from build123d import *

# Parameters (mm, degrees)
F0_R     = 1
F1_DEPTH = 8.3
F2_SIZE  = 0.5


with BuildPart() as f1:
    # F0 (on Top) → F1 (new body)
    with BuildSketch(Plane.XY):
        with BuildLine():
            Line((3.666061, 3.4), (-3.666061, 3.4))
            ThreePointArc((-3.666061, 3.4), (-5, 0), (-3.666061, -3.4))
            Line((-3.666061, -3.4), (3.666061, -3.4))
            ThreePointArc((3.666061, -3.4), (5, 0), (3.666061, 3.4))
        make_face()
        Circle(F0_R, mode=Mode.SUBTRACT)
    extrude(amount=F1_DEPTH)

    # F2
    f2_edges = [f1.edges().sort_by_distance(p)[0] for p in [
        (-5, 0, 0),
        (0, -3.4, 0),
        (5, 0, 0),
        (0, 3.4, 0),
        (-1, 0, 0),
    ]]
    chamfer(f2_edges, length=F2_SIZE)


solid = f1.part
Could you check a few things on this model? Use its own coordinates, in mm. Round coordinates to 2 decimals unless told otherwise and drop trailing zeros. Write each loop counter-clockwise with the first axis right and the second up, starting at its lowest first coordinate (ties: lowest second). Pieces come first, ordered by that corner, then holes. Notation, with made-up numbers: (-33.75, 70) - (-10.75, 70) arc R17 ccw to (-10.75, 95) - close; hole circle Ø2 at (-9, 55.25). An arc over 180 degrees is marked (long way). Put each result on its own line as item: value. Start each with the question number.
(1) I want a section at A-A, the plane y = 0. Please give me the cut outline in (x, z), plus the area to 3 significant figures.
(2) Will these pins go through, and if not, where does the flat tip stop? pin 1 (2 mm diameter, centred on y = 2, z = 2.5, fed in from +X); pin 2 (1.8 mm diameter, centred on x = 0, y = 0, fed in from -Z); pin 3 (4 mm diameter, centred on x = 1, y = -0.5, fed in from -Z).
(3) I need wall thicknesses on probe 1 along Y at (x, z) = (0, 1); probe 2 along X at (y, z) = (0.75, 7.25); probe 3 along X at (y, z) = (-1.75, 1.5). Which ranges of each line are inside material? Lowest first, please.
(4) Thinking about a two-plate mould opening in Y: for faces 1 (the flat face through (-1.1, 1.3, 0)), 2 (the cylindrical face through (0, -1, 4)), 3 (the conical face through (4.64, -0.05, 0.14)), which applies, released by +Y, released by -Y, zero draft, split by the parting line, or undercut?
(5) I want a section at B-B, the plane x = 0. Please give me the cut outline in (y, z).
(6) I want a section at C-C, the plane z = 3.75. Please give me the cut outline in (x, y).
Here are the results:
1. outline: (-5, 0.5) - (-4.5, 0) - (-1.5, 0) - (-1, 0.5) - (-1, 8.3) - (-5, 8.3) - close; (1, 0.5) - (1.5, 0) - (4.5, 0) - (5, 0.5) - (5, 8.3) - (1, 8.3) - close
1. area: 65.9 mm^2
2. pin 1: stops at x = 4.9
2. pin 2: passes through
2. pin 3: stops at z = 0
3. probe 1: y = -3.4 to -1, 1 to 3.4
3. probe 2: x = -4.94 to -0.66, 0.66 to 4.94
3. probe 3: x = -4.68 to 4.68
4. face 1: zero draft
4. face 2: undercut
4. face 3: split by the parting line
5. outline: (-3.4, 0.5) - (-2.9, 0) - (-1.5, 0) - (-1, 0.5) - (-1, 8.3) - (-3.4, 8.3) - close; (1, 0.5) - (1.5, 0) - (2.9, 0) - (3.4, 0.5) - (3.4, 8.3) - (1, 8.3) - close
6. outline: (-3.67, -3.4) - (3.67, -3.4) arc R5 ccw to (3.67, 3.4) - (-3.67, 3.4) arc R5 ccw to start; hole circle Ø2 at (0, 0)
